For this review, take the finished solid that the model builds, in its own axes (mm). Face numbers are marked on the shaded views. Coordinates: 2 decimals unless noted, no trailing zeros. Write each loop counter-clockwise with the first axis right and the second up, starting at its lowest first coordinate (ties: lowest second). Pieces come first, ordered by that corner, then holes.
1) Insertion check: P1, Ø1, axis at x = -1, y = -4, coming from the -Z side; P2, Ø0.6, axis at x = -1, y = -3, coming from the +Z side; P3, Ø2, axis at x = -1.5, z = 64, coming from the -Y side. Each pin has a flat end and moves straight along its axis. Give the tip position at first contact, or say it passes through.
2) We need section B-B on x = 21. Write out the cut boundary in (y, z), then the cut area to 3 significant figures.
3) We need section C-C on x = 9.5. Write out the cut boundary in (y, z).
4) Mouldability with a two-part tool opening along X and no side actions: class the marked faces 1 and 2 as pulls with the +X half, pulls with the -X half, needs draft (parallel to the pull), parting line crosses it, or undercut.
5) We need section D-D on z = 66. Write out the cut boundary in (x, y).
6) To check wall thickness, follow line 1 along Z through (x, y) = (18, 0.2); line 2 along Z through (x, y) = (38.5, 0.55); line 3 along X through (y, z) = (-3.25, 27.5). State the ranges of each line that lie inside material, in increasing order.
7) We need section A-A on z = 39.5. Write out the cut boundary in (x, y), then the cut area to 3 significant figures.
from build123d import *

# Parameters (mm, degrees)
EXTRUDE_4_DEPTH          = 1
EXTRUDE_START            = -5
EXTRUDE_5_DEPTH          = 5
CUT_EXTRUDE_START        = 5
CUT_EXTRUDE_1_DEPTH      = 1
CUT_EXTRUDE_2_DEPTH      = 116.376685757
CUT_EXTRUDE_2_DEPTH_BACK = 116.376685757
SKETCH_8_W               = 22
SKETCH_8_H               = 6
SKETCH_8_W_2             = 75
SKETCH_8_H_2             = 57
CUT_EXTRUDE_3_REACH      = 118.919
SKETCH_9_W               = 10
SKETCH_9_H               = 3


with BuildPart() as part:
    # Эскиз1 → Бобышка-Вытянуть4 (new body)
    with BuildSketch(Plane(origin=(0, 0, 0), x_dir=(1, 0, 0), z_dir=(0, 1, 0))):
        with BuildLine():
            Line((-2.084374602, -1.449446306), (-2.084374602, -72.949446306))
            ThreePointArc((-2.084374602, -72.949446306), (-0.619908508, -76.484980212), (2.915625398, -77.949446306))
            Line((2.915625398, -77.949446306), (79.915625398, -77.949446306))
            ThreePointArc((79.915625398, -77.949446306), (83.451159304, -76.484980212), (84.915625398, -72.949446306))
            Line((84.915625398, -72.949446306), (84.915625398, -1.449446306))
            ThreePointArc((84.915625398, -1.449446306), (83.451159304, 2.0860876), (79.915625398, 3.550553694))
            Line((79.915625398, 3.550553694), (2.915625398, 3.550553694))
            ThreePointArc((2.915625398, 3.550553694), (-0.619908508, 2.0860876), (-2.084374602, -1.449446306))
        make_face()
    extrude(amount=EXTRUDE_4_DEPTH)

    # Эскиз1<14> → Бобышка-Вытянуть5 (add)
    with BuildSketch(Plane(origin=(0, 0, 0), x_dir=(1, 0, 0), z_dir=(0, 1, 0)).offset(EXTRUDE_START)):
        with BuildLine():
            Line((2.915625398, 3.550553694), (79.915625398, 3.550553694))
            ThreePointArc((79.915625398, 3.550553694), (83.451159304, 2.0860876), (84.915625398, -1.449446306))
            Line((84.915625398, -1.449446306), (84.915625398, -72.949446306))
            ThreePointArc((84.915625398, -72.949446306), (83.451159304, -76.484980212), (79.915625398, -77.949446306))
            Line((79.915625398, -77.949446306), (2.915625398, -77.949446306))
            ThreePointArc((2.915625398, -77.949446306), (-0.619908508, -76.484980212), (-2.084374602, -72.949446306))
            Line((-2.084374602, -72.949446306), (-2.084374602, -1.449446306))
            ThreePointArc((-2.084374602, -1.449446306), (-0.619908508, 2.0860876), (2.915625398, 3.550553694))
        make_face()
        with BuildLine():
            ThreePointArc((2.915625398, 1.550553694), (0.794305055, 0.671874038), (-0.084374602, -1.449446306))
            Line((-0.084374602, -1.449446306), (-0.084374602, -72.949446306))
            ThreePointArc((-0.084374602, -72.949446306), (0.794305055, -75.070766649), (2.915625398, -75.949446306))
            Line((2.915625398, -75.949446306), (79.915625398, -75.949446306))
            ThreePointArc((79.915625398, -75.949446306), (82.036945742, -75.070766649), (82.915625398, -72.949446306))
            Line((82.915625398, -72.949446306), (82.915625398, -1.449446306))
            ThreePointArc((82.915625398, -1.449446306), (82.036945742, 0.671874038), (79.915625398, 1.550553694))
            Line((79.915625398, 1.550553694), (2.915625398, 1.550553694))
        make_face(mode=Mode.SUBTRACT)
    extrude(amount=EXTRUDE_5_DEPTH)

    # Эскиз3 → Вырез-Вытянуть1 (cut)
    with BuildSketch(Plane.XZ.offset(CUT_EXTRUDE_START)):
        with BuildLine():
            Line((2.915625398, -2.550553694), (79.915625398, -2.550553694))
            ThreePointArc((79.915625398, -2.550553694), (82.744052523, -1.378980819), (83.915625398, 1.449446306))
            Line((83.915625398, 1.449446306), (83.915625398, 72.949446306))
            ThreePointArc((83.915625398, 72.949446306), (82.744052523, 75.777873431), (79.915625398, 76.949446306))
            Line((79.915625398, 76.949446306), (2.915625398, 76.949446306))
            ThreePointArc((2.915625398, 76.949446306), (0.087198273, 75.777873431), (-1.084374602, 72.949446306))
            Line((-1.084374602, 72.949446306), (-1.084374602, 1.449446306))
            ThreePointArc((-1.084374602, 1.449446306), (0.087198273, -1.378980819), (2.915625398, -2.550553694))
        make_face()
    extrude(amount=-CUT_EXTRUDE_1_DEPTH, mode=Mode.SUBTRACT)

    # Эскиз8 → Вырез-Вытянуть2 (cut, two sides: drawn at the far end of the back side and taken through both)
    with BuildSketch(Plane.XZ.offset(-CUT_EXTRUDE_2_DEPTH_BACK)):
        with BuildLine():
            Line((40.415625398, 55.949446306), (80.415625398, 55.949446306))
            ThreePointArc((80.415625398, 55.949446306), (81.829838961, 56.535232743), (82.415625398, 57.949446306))
            Line((82.415625398, 57.949446306), (82.415625398, 73.449446306))
            ThreePointArc((82.415625398, 73.449446306), (81.829838961, 74.863659868), (80.415625398, 75.449446306))
            Line((80.415625398, 75.449446306), (42.415625398, 75.449446306))
            ThreePointArc((42.415625398, 75.449446306), (41.001411836, 74.863659868), (40.415625398, 73.449446306))
            Line((40.415625398, 73.449446306), (40.415625398, 55.949446306))
        make_face()
        with Locations((25.915625398, 65.949446306)):
            Rectangle(SKETCH_8_W, SKETCH_8_H)
        with Locations((41.415625398, 27.449446306)):
            Rectangle(SKETCH_8_W_2, SKETCH_8_H_2)
    extrude(amount=CUT_EXTRUDE_2_DEPTH + CUT_EXTRUDE_2_DEPTH_BACK, mode=Mode.SUBTRACT)

    # Эскиз9 → Вырез-Вытянуть3 (cut, up to next)
    with BuildSketch(Plane.ZY.offset(2.084374602), mode=Mode.PRIVATE) as cut_extrude_3_sk1:
        with Locations((64.949446306, -3.5)):
            Rectangle(SKETCH_9_W, SKETCH_9_H)
    cut_extrude_3_tool1 = extrude(cut_extrude_3_sk1.sketch, amount=-CUT_EXTRUDE_3_REACH, mode=Mode.PRIVATE) & part.part
    add(cut_extrude_3_tool1.solids().sort_by_distance((-2.084375, -3.5, 64.949446))[0], mode=Mode.SUBTRACT)


solid = part.part
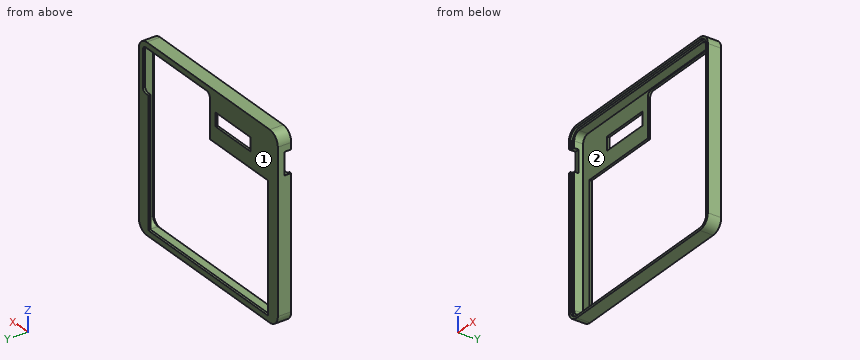
Result:
1. P1: stops at z = -2.2
1. P2: stops at z = 76.4
1. P3: stops at y = -2
2. outline: (-5, -3.55) - (1, -3.55) - (1, -1.05) - (0, -1.05) - (0, -1.55) - (-4, -1.55) - (-4, -2.55) - (-5, -2.55) - close; (-5, 76.95) - (-4, 76.95) - (-4, 75.95) - (0, 75.95) - (0, 68.95) - (1, 68.95) - (1, 77.95) - (-5, 77.95) - close; (0, 55.95) - (1, 55.95) - (1, 62.95) - (0, 62.95) - close
2. area: 36.5 mm2
3. outline: (-5, -3.55) - (1, -3.55) - (1, -1.05) - (0, -1.05) - (0, -1.55) - (-4, -1.55) - (-4, -2.55) - (-5, -2.55) - close; (-5, 76.95) - (-4, 76.95) - (-4, 75.95) - (0, 75.95) - (0, 55.95) - (1, 55.95) - (1, 77.95) - (-5, 77.95) - close
4. face 1: needs draft
4. face 2: undercut
5. outline: (-2.08, -2) - (-0.08, -2) - (-0.08, 0) - (14.92, 0) - (14.92, 1) - (-2.08, 1) - close; (36.92, 0) - (40.42, 0) - (40.42, 1) - (36.92, 1) - close; (82.42, 0) - (82.92, 0) - (82.92, -4) - (83.92, -4) - (83.92, -5) - (84.92, -5) - (84.92, 1) - (82.42, 1) - close
6. line 1: z = -3.55 to -1.05, 55.95 to 62.95, 68.95 to 77.95
6. line 2: z = -3.55 to -1.05, 55.95 to 77.95
6. line 3: x = -2.08 to -0.08, 82.92 to 84.92
7. outline: (-2.08, -5) - (-1.08, -5) - (-1.08, -4) - (-0.08, -4) - (-0.08, 0) - (3.92, 0) - (3.92, 1) - (-2.08, 1) - close; (78.92, 0) - (82.92, 0) - (82.92, -4) - (83.92, -4) - (83.92, -5) - (84.92, -5) - (84.92, 1) - (78.92, 1) - close
7. area: 30.0 mm2
